Model file for the job. Use its own axes, mm. Give positions to 0.01 mm unless a question says otherwise; leave off trailing zeros. Loops run counter-clockwise (first coordinate to the right, second up) from the corner with the lowest first, then second, coordinate; pieces in that order, holes last. Notation, with made-up numbers: (-1.5, -20) - (13.5, -20) arc R24 ccw to (13.5, -6) - close; hole circle Ø11 at (-39, -3.5). An arc over 180 degrees is marked (long way). Answer as CSV lines item,"result". Start each with the question number.
Item 1: Saw through at B-B on y = 0. Give the cut face in (x, z) (1 decimal).
Item 2: Saw through at C-C on x = 20. Give the cut face in (y, z), plus the area to 3 significant figures.
Item 3: Pull direction X, two halves, no side cores. Call faces 1 (the cylindrical face through (11.117, 0.209, 1.507)), 2 (the flat face through (0, 10.319, 1)), 3 (the cylindrical face through (-33.114, 8.409, 1.507)): pulls with the +X half, pulls with the -X half, needs draft (parallel to the pull), parting line crosses it, or undercut.
Item 4: Saw through at A-A on z = 1.9. State how many separate pieces and enclosed holes the cut face has, plus the area to 3 significant figures.
Item 5: Saw through at D-D on y = -7.25. Give the cut face in (x, z).
Item 6: Pin check, flat tips, straight feed: pin 1 (5.5 mm diameter, centred on x = 28.58, y = -3.97, fed in from +Z); pin 2 (4.5 mm diameter, centred on x = 28.58, y = 3.97, fed in from -Z). Stop position of each tip, or through.
Item 7: Drill centre lines: L1, parallel to Y at x = 18.5, z = 2.75; L2, parallel to X at y = 5.75, z = 2.4; L3, parallel to Y at x = 27.5, z = 1.7. Where is each one in solid material? Low to high. Write a range as from..to.
from build123d import *

# Parameters (mm, degrees)
SKETCH1_W           = 69.85
SKETCH1_H           = 20.6375
SKETCH1_R           = 2.38125
BOSS_EXTRUDE1_DEPTH = 2.9718
FILLET1_R           = 6.35
SKETCH2_R           = 4.7625
CUT_EXTRUDE1_DEPTH  = 3.9718


with BuildPart() as part:
    # Sketch1 → Boss-Extrude1 (new body)
    with BuildSketch(Plane.XY):
        Rectangle(SKETCH1_W, SKETCH1_H)
        with Locations((-28.575, 3.96875)):
            Circle(SKETCH1_R, mode=Mode.SUBTRACT)
        with Locations((-28.575, -3.96875)):
            Circle(SKETCH1_R, mode=Mode.SUBTRACT)
        with Locations((28.575, 3.96875)):
            Circle(SKETCH1_R, mode=Mode.SUBTRACT)
        with Locations((28.575, -3.96875)):
            Circle(SKETCH1_R, mode=Mode.SUBTRACT)
    extrude(amount=BOSS_EXTRUDE1_DEPTH)

    # Fillet1
    fillet1_edges = [part.edges().sort_by_distance(p)[0] for p in [
        (-34.925, 10.31875, 1.4859),
        (34.925, 10.31875, 1.4859),
        (34.925, -10.31875, 1.4859),
        (-34.925, -10.31875, 1.4859),
    ]]
    fillet(fillet1_edges, radius=FILLET1_R)

    # Sketch2 → Cut-Extrude1 (cut, through all)
    with BuildSketch(Plane.XY.offset(2.9718)):
        with Locations((15.875, 0)):
            Circle(SKETCH2_R)
    extrude(amount=-CUT_EXTRUDE1_DEPTH, mode=Mode.SUBTRACT)


solid = part.part
Responses:
1,outline,"(-34.9, 0) - (11.1, 0) - (11.1, 3) - (-34.9, 3) - close; (20.6, 0) - (34.9, 0) - (34.9, 3) - (20.6, 3) - close"
2,outline,"(-10.32, 0) - (-2.38, 0) - (-2.38, 2.97) - (-10.32, 2.97) - close; (2.38, 0) - (10.32, 0) - (10.32, 2.97) - (2.38, 2.97) - close"
2,area,"47.2 mm2"
3,face 1,"undercut"
3,face 2,"needs draft"
3,face 3,"pulls with the -X half"
4,separate pieces,"1"
4,enclosed holes,"5"
4,area,"1,260 mm2"
5,outline,"(-34.01, 0) - (34.01, 0) - (34.01, 2.97) - (-34.01, 2.97) - close"
6,pin 1,"z = 2.97"
6,pin 2,"through"
7,L1,"-10.32..-3.97, 3.97..10.32"
7,L2,"-34.67..-30.16, -26.99..26.99, 30.16..34.67"
7,L3,"-10.32..-6.09, -1.84..1.84, 6.09..10.32"
